Print and shaded views of the part. All mm, measured from the part's lowest x, y and z. A direction names the side the tool comes from. Coordinates: 2 decimals unless noted, no trailing zeros. Loops run counter-clockwise (first coordinate to the right, second up) from the corner with the lowest first, then second, coordinate; pieces in that order, holes last.
1) Two-plate mould, pull along Y, no slides. Class the marked faces 1, 2 and 3: +Y half, -Y half, draft (parallel to the pull), parting line (faces both ways), or undercut.
2) Which spindle directions (+Z, -Z, +X, -X, +Y, -Y) get a long thin tool onto all of the face, cutting with end or side? Do the marked faces 4 and 5. Say none if no direction does.
3) Saw through at C-C, the plane x = 30.5. Write the cut outline in (y, z), and give its area (3 significant figures).
4) Saw through at D-D, the plane y = 36.5. Write the cut outline in (x, z).
5) Wall check: line 1 along Y through (x, z) = (37.7, 18); line 2 along Y through (x, z) = (33.15, 18); line 3 along Z through (x, y) = (11, 42.5). Give the ranges that are in metal, low to high.
6) Saw through at A-A, the plane y = 71. Write the cut outline in (x, z).
7) Pin check, flat tips, straight feed: pin 1 Ø1 at (x, z) = (28, 28.5) entering from +Y; pin 2 Ø3 at (x, z) = (34.5, 20) entering from -Y; pin 3 Ø12 at (y, z) = (10, 29.5) entering from -X. Stop position of each tip, or through.
8) Saw through at B-B, the plane z = 18. Write the cut outline in (x, y).
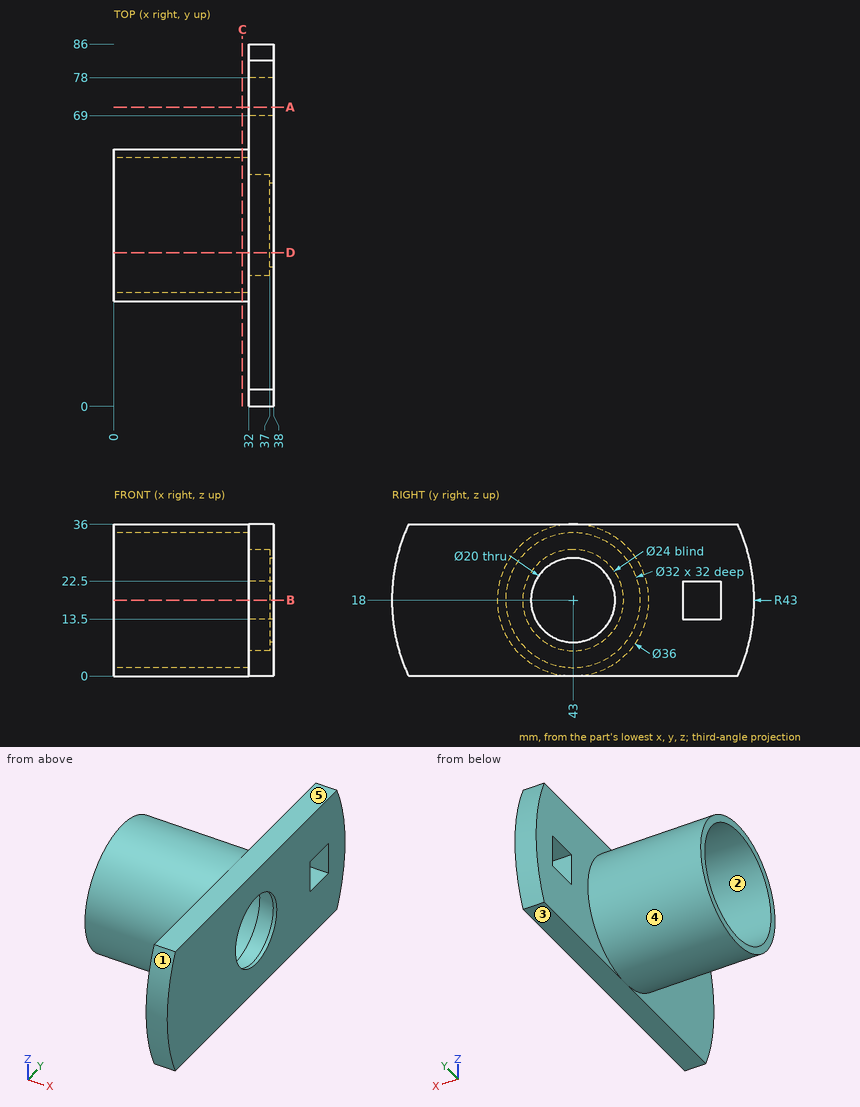
Data:
1. face 1: -Y half
1. face 2: undercut
1. face 3: draft
2. face 4: -X
2. face 5: +Z, +X, -X, +Y, -Y
3. outline: circle Ø36 at (43, 18); hole circle Ø32 at (43, 18)
3. area: 214 mm2
4. outline: (0, 1.21) - (32, 1.21) - (32, 0) - (38, 0) - (38, 10.4) - (37, 10.4) - (37, 7.91) - (32, 7.91) - (32, 3.38) - (0, 3.38) - close; (0, 32.62) - (32, 32.62) - (32, 28.09) - (37, 28.09) - (37, 25.6) - (38, 25.6) - (38, 36) - (32, 36) - (32, 34.79) - (0, 34.79) - close
5. line 1: y = 0 to 33, 53 to 69, 78 to 86
5. line 2: y = 0 to 31, 55 to 69, 78 to 86
5. line 3: z = 0.01 to 2.01, 33.99 to 35.99
6. outline: (32, 0) - (38, 0) - (38, 13.5) - (32, 13.5) - close; (32, 22.5) - (38, 22.5) - (38, 36) - (32, 36) - close
7. pin 1: stops at y = 57.97
7. pin 2: stops at y = 0
7. pin 3: stops at x = 32
8. outline: (0, 25) - (32, 25) - (32, 0) - (38, 0) - (38, 33) - (37, 33) - (37, 31) - (32, 31) - (32, 27) - (0, 27) - close; (0, 59) - (32, 59) - (32, 55) - (37, 55) - (37, 53) - (38, 53) - (38, 69) - (32, 69) - (32, 61) - (0, 61) - close; (32, 78) - (38, 78) - (38, 86) - (32, 86) - close
